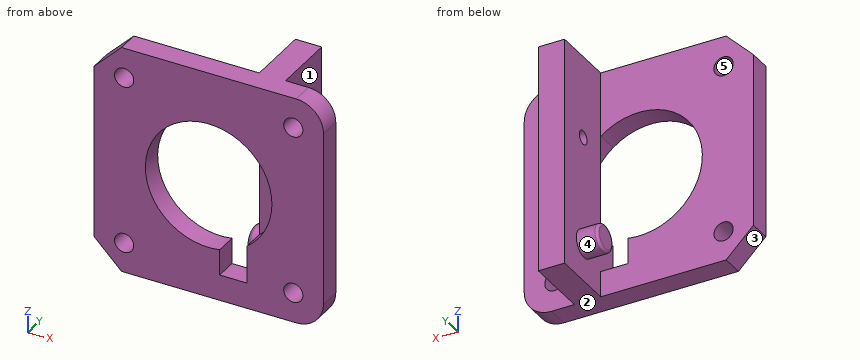
```python
from build123d import *

# Parameters (mm, degrees)
SKETCH2_W           = 42
SKETCH2_H           = 42.01
BOSS_EXTRUDE2_DEPTH = 4.02
SKETCH3_W           = 4.82
SKETCH3_H           = 15.81
BOSS_EXTRUDE3_DEPTH = 42.01
SKETCH4_R           = 11.6
CUT_EXTRUDE1_DEPTH  = 4.02
SKETCH5_R           = 1.255
CUT_EXTRUDE2_DEPTH  = 33.803184685
CHAMFER1_SIZE       = 5
SKETCH6_R           = 1.76
CUT_EXTRUDE3_DEPTH  = 4.02
FILLET1_R           = 5
SKETCH7_R           = 2.515
BOSS_EXTRUDE4_DEPTH = 3.92
FILLET3_R           = 0.5


with BuildPart() as part:
    # Sketch2 → Boss-Extrude2 (new body)
    with BuildSketch(Plane(origin=(0, 0, 0), x_dir=(1, 0, 0), z_dir=(0, 1, 0))):
        with Locations((0.04, -0.105)):
            Rectangle(SKETCH2_W, SKETCH2_H)
        with BuildLine():
            Line((2.023352998, 16.161086645), (2.023352998, 11.422173289))
            ThreePointArc((2.023352998, 11.422173289), (-7.967970915, -8.430387861), (11.29, 2.663813057))
            Line((11.29, 2.663813057), (11.29, 16.161086645))
            Line((11.29, 16.161086645), (4.04, 16.161086645))
            Line((4.04, 16.161086645), (2.023352998, 16.161086645))
        make_face(mode=Mode.SUBTRACT)
    extrude(amount=BOSS_EXTRUDE2_DEPTH)

    # Sketch3 → Boss-Extrude3 (add)
    with BuildSketch(Plane.XY.offset(21.11)):
        with Locations((9.433184685, 7.905)):
            Rectangle(SKETCH3_W, SKETCH3_H)
    extrude(amount=-BOSS_EXTRUDE3_DEPTH)

    # Sketch4 → Cut-Extrude1 (cut)
    with BuildSketch(Plane.XZ):
        Circle(SKETCH4_R)
    extrude(amount=-CUT_EXTRUDE1_DEPTH, mode=Mode.SUBTRACT)

    # Sketch5 → Cut-Extrude2 (cut, through all)
    with BuildSketch(Plane(origin=(11.843184685, 0, 0), x_dir=(0, 0, -1), z_dir=(1, 0, 0))):
        with Locations((-5.905, 9.751921695)):
            Circle(SKETCH5_R)
    extrude(amount=-CUT_EXTRUDE2_DEPTH, mode=Mode.SUBTRACT)

    # Chamfer1
    chamfer1_edges = [part.edges().sort_by_distance(p)[0] for p in [
        (-20.96, 2.01, -20.9),
        (-20.96, 2.01, 21.11),
    ]]
    chamfer(chamfer1_edges, length=CHAMFER1_SIZE)

    # Sketch6 → Cut-Extrude3 (cut)
    with BuildSketch(Plane(origin=(0, 4.02, 0), x_dir=(1, 0, 0), z_dir=(0, 1, 0))):
        with Locations((-15.48, 15.42)):
            Circle(SKETCH6_R)
        with Locations((15.52, 15.42)):
            Circle(SKETCH6_R)
        with Locations((-15.48, -15.585900263)):
            Circle(SKETCH6_R)
        with Locations((15.52, -15.585900263)):
            Circle(SKETCH6_R)
    extrude(amount=-CUT_EXTRUDE3_DEPTH, mode=Mode.SUBTRACT)

    # Fillet1
    fillet1_edges = [part.edges().sort_by_distance(p)[0] for p in [
        (21.04, 2.01, -20.9),
        (21.04, 2.01, 21.11),
    ]]
    fillet(fillet1_edges, radius=FILLET1_R)

    # Sketch7 → Boss-Extrude4 (add)
    with BuildSketch(Plane.ZY.offset(-7.023184685)):
        with Locations((-13.936978862, 9.480319198)):
            Circle(SKETCH7_R)
    extrude(amount=BOSS_EXTRUDE4_DEPTH)

    # Fillet3
    fillet3_edges = [part.edges().sort_by_distance(p)[0] for p in [
        (3.103184685, 9.480319198, -16.451978862),
    ]]
    fillet(fillet3_edges, radius=FILLET3_R)


solid = part.part
```
Geometry: final body of the model. Coordinates: model frame, mm. Face numbers are marked on the shaded views. A direction names the side the tool comes from. Coordinates: 2 decimals unless noted, no trailing zeros. Loops run counter-clockwise (first coordinate to the right, second up) from the corner with the lowest first, then second, coordinate; pieces in that order, holes last. Notation, with made-up numbers: M 82.25,21.25 L 97.25,21.25 A16 ccw 97.25,48.25 Z; hole C -21,23.25 d11. An arc over 180 degrees is marked long. Put each result on its own line as item: value.
(1) Cut plane B-B on z = 8. Return the cut outline in (x, y), then the cut area to 3 significant figures.
Answer sheet:
outline: M -20.96,0 L -8.4,0 L -8.4,4.02 L -20.96,4.02 Z; M 7.02,4.02 L 8.4,4.02 L 8.4,0 L 21.04,0 L 21.04,4.02 L 11.84,4.02 L 11.84,15.81 L 7.02,15.81 Z
area: 158 mm^2
(2) Access query for the marked faces 1 and 2. Directions: +Z, -Z, +X, -X, +Y, -Y. A direction counts if a zero-diameter tool reaches every point of the face in a straight line with its end or side. Return the directions, or none.
Answer sheet:
face 1: +Z, -Z, +X, +Y
face 2: -Z, +X, -X, +Y, -Y
(3) Cut plane A-A on x = 0. Return the cut outline in (y, z), then the cut area to 3 significant figures.
Answer sheet:
outline: M 0,-20.9 L 4.02,-20.9 L 4.02,-11.6 L 0,-11.6 Z; M 0,11.6 L 4.02,11.6 L 4.02,21.11 L 0,21.11 Z
area: 75.6 mm^2
(4) Cut plane C-C on x = 15.52. Return the cut outline in (y, z), then the cut area to 3 significant figures.
Answer sheet:
outline: M 0,-20.9 L 4.02,-20.9 L 4.02,-17.18 L 0,-17.18 Z; M 0,-13.66 L 4.02,-13.66 L 4.02,13.83 L 0,13.83 Z; M 0,17.35 L 4.02,17.35 L 4.02,21.11 L 0,21.11 Z
area: 141 mm^2
(5) Cut plane D-D on z = 0. Return the cut outline in (x, y), then the cut area to 3 significant figures.
Answer sheet:
outline: M -20.96,0 L -11.6,0 L -11.6,4.02 L -20.96,4.02 Z; M 7.02,4.02 L 11.6,4.02 L 11.6,0 L 21.04,0 L 21.04,4.02 L 11.84,4.02 L 11.84,15.81 L 7.02,15.81 Z
area: 132 mm^2
(6) Material intervals for probe 1 along Z at (x, y) = (15.52, 2.3); probe 2 along X at (y, z) = (1.45, -15.42); probe 3 along Z at (x, y) = (17, 2.25), sorted ascending.
Answer sheet:
probe 1: z = -20.9 to -17.18, -13.66 to 13.83, 17.35 to 21.11
probe 2: x = -20.96 to -17.24, -13.72 to 2.02, 7.02 to 13.76, 17.28 to 21.04
probe 3: z = -20.81 to -16.37, -14.47 to 14.63, 16.54 to 21.02
(7) Draft query along X for the marked faces 3, 4 and 5. Return one class per face: pulls with the +X half, pulls with the -X half, needs draft (parallel to the pull), parting line crosses it, or undercut.
Answer sheet:
face 3: pulls with the -X half
face 4: needs draft
face 5: undercut
(8) First-contact query: pin 1 (6 mm diameter, centred on y = 9.5, z = -12, fed in from +X); pin 2 (4.5 mm diameter, centred on y = 9, z = -14, fed in from -X); pin 3 (3 mm diameter, centred on y = 9.75, z = 5.9, fed in from -X). Flat tips, straight axial feed; report the tip coordinate or a pass-through.
Answer sheet:
pin 1: stops at x = 11.84
pin 2: stops at x = 3.1
pin 3: stops at x = 7.02
